CAD build for the part. Positions are in the model's coordinates, mm. Face numbers are marked on the shaded views. Round coordinates to 2 decimals unless told otherwise and drop trailing zeros. Loops run counter-clockwise (first coordinate to the right, second up) from the corner with the lowest first, then second, coordinate; pieces in that order, holes last.
```python
from build123d import *

# Parameters (mm, degrees)
SKETCH1_R           = 3
BOSS_EXTRUDE6_DEPTH = 3


with BuildPart() as part:
    # Sketch1 → Boss-Extrude6 (new body)
    with BuildSketch(Plane(origin=(0, 0, 0), x_dir=(1, 0, 0), z_dir=(0, 1, 0))):
        with BuildLine():
            ThreePointArc((70, 35), (107.5, 72.5), (145, 35))
            Line((145, 35), (145, 8))
            Line((145, 8), (105, 8))
            Line((105, 8), (105, 5))
            Line((105, 5), (145, 5))
            Line((145, 5), (145, 0))
            Line((145, 0), (70, 0))
            Line((70, 0), (70, 35))
        make_face()
        with Locations((107.5, 35)):
            Circle(SKETCH1_R, mode=Mode.SUBTRACT)
        Polygon((87.5, 10.989200562), (87.5, 20.989200562), (87.5, 30.989200562), (84.5, 30.989200562), (84.5, 10.989200562), align=None, mode=Mode.SUBTRACT)
        Polygon((130.5, 10.989200562), (127.5, 10.989200562), (127.5, 20.989200562), (127.5, 30.989200562), (130.5, 30.989200562), align=None, mode=Mode.SUBTRACT)
    extrude(amount=BOSS_EXTRUDE6_DEPTH)


solid = part.part
```
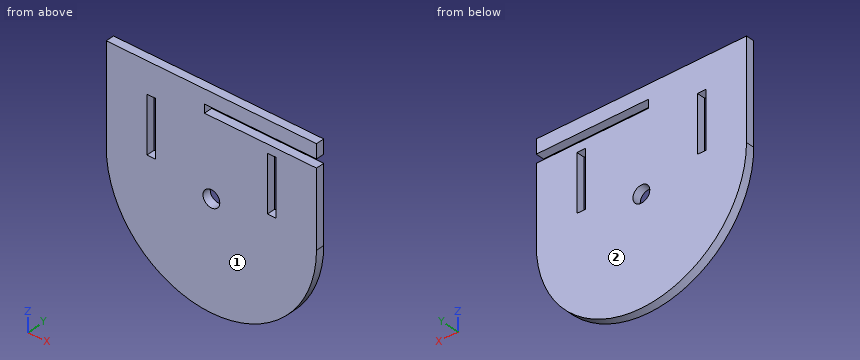
Item 1: Cut at C-C, the plane x = 107.5. Give the cut face in (y, z).
Answers follow:
outline: (0, -72.5) - (3, -72.5) - (3, -38) - (0, -38) - close; (0, -32) - (3, -32) - (3, -8) - (0, -8) - close; (0, -5) - (3, -5) - (3, 0) - (0, 0) - close
Item 2: Two-plate mould, pull along Y, no slides. Class the marked faces 1 and 2: released by +Y, released by -Y, zero draft, split by the parting line, or undercut.
Answers follow:
face 1: released by -Y
face 2: released by +Y
Item 3: Cut at A-A, the plane x = 137.5. Give the cut face in (y, z), plus the area to 4 significant figures.
Answers follow:
outline: (0, -57.5) - (3, -57.5) - (3, -8) - (0, -8) - close; (0, -5) - (3, -5) - (3, 0) - (0, 0) - close
area: 163.5 mm2
Item 4: Cut at B-B, the plane y = 2.4. Give the cut face in (x, z).
Answers follow:
outline: (70, -35) arc R37.5 ccw to (145, -35) - (145, -8) - (105, -8) - (105, -5) - (145, -5) - (145, 0) - (70, 0) - close; hole (84.5, -30.99) - (87.5, -30.99) - (87.5, -10.99) - (84.5, -10.99) - close; hole circle Ø6 at (107.5, -35); hole (127.5, -30.99) - (130.5, -30.99) - (130.5, -10.99) - (127.5, -10.99) - close
Item 5: Flat gauge pins, fed straight in: P1, Ø5, axis at x = 107.5, z = -35, coming from the -Y side; P2, Ø1.5, axis at x = 120, y = 2.5, coming from the -Z side; P3, Ø1.5, axis at x = 130, y = 1, coming from the -Z side; P4, Ø0.9, axis at y = 1.5, z = -6, coming from the +X side. Where does each tip first touch, or does it go through?
Answers follow:
P1: passes through
P2: stops at z = -70.61
P3: stops at z = -65.55
P4: stops at x = 105
Item 6: Probe line 1 (Z direction, x = 107.5, y = 0.7); line 2 (X direction, y = 2.55, z = -23); line 3 (X direction, y = 0.8, z = -35). List the from-to ranges inside material, lowest first.
Answers follow:
line 1: z = -72.5 to -38, -32 to -8, -5 to 0
line 2: x = 70 to 84.5, 87.5 to 127.5, 130.5 to 145
line 3: x = 70 to 104.5, 110.5 to 145
Item 7: Cut at D-D, the plane z = -56. Give the cut face in (x, y).
Answers follow:
outline: (76.43, 0) - (138.57, 0) - (138.57, 3) - (76.43, 3) - close
